```python
from build123d import *

# Parameters (mm, degrees)
SKETCH1_W                      = 15
SKETCH1_H                      = 5.8
CBORE_FOR_M3_SHCS1_D           = 3.2
CBORE_FOR_M3_SHCS1_CBORE_D     = 8
CBORE_FOR_M3_SHCS1_CBORE_DEPTH = 4.3
FILLET2_R                      = 4
FILLET3_R                      = 1


with BuildPart() as part:
    # Sketch1 → Revolve1 (revolve)
    with BuildSketch(Plane.XY, mode=Mode.PRIVATE) as revolve1_sk:
        with Locations((7.5, -2.9)):
            Rectangle(SKETCH1_W, SKETCH1_H)
    revolve(revolve1_sk.sketch.rotate(Axis((0, 0, 0), (0, -1, 0)), 180), axis=Axis((0, 0, 0), (0, -1, 0)))

    # CBORE for M3 SHCS1 (through all)
    with Locations(Plane(origin=(0, -5.8, 0), x_dir=(-1, 0, 0), z_dir=(0, -1, 0))):
        with Locations((0, 0)):
            CounterBoreHole(CBORE_FOR_M3_SHCS1_D / 2, CBORE_FOR_M3_SHCS1_CBORE_D / 2, CBORE_FOR_M3_SHCS1_CBORE_DEPTH)

    # Fillet2
    fillet2_edges = [part.edges().sort_by_distance(p)[0] for p in [
        (15, -5.8, 0),
    ]]
    fillet(fillet2_edges, radius=FILLET2_R)

    # Fillet3
    fillet3_edges = [part.edges().sort_by_distance(p)[0] for p in [
        (4, -5.8, 0),
    ]]
    fillet(fillet3_edges, radius=FILLET3_R)


solid = part.part
```
For this review, take the finished solid that the model builds, in its own axes (mm). A direction names the side the tool comes from. Coordinates: 2 decimals unless noted, no trailing zeros. Write each loop counter-clockwise with the first axis right and the second up, starting at its lowest first coordinate (ties: lowest second). Pieces come first, ordered by that corner, then holes. Notation, with made-up numbers: (19.25, 76.5) - (71.25, 76.5) arc R30 cw to (71.25, 103.5) - close; hole circle Ø4 at (89.25, -26). An arc over 180 degrees is marked (long way). Answer in a Markdown table with one row per item. Add a question column.
Q1. Tool access review of faces 1 (the flat face through (5, -5.8, 2)), 2 (the cylindrical face through (0.867, -3.173, 3.905)): name each direction out of +Z, -Z, +X, -X, +Y, -Y from which nothing blocks a thin tool from reaching the whole face with its end or side.
Q2. Draft analysis for pull direction Z (two halves, no side actions). For faces 3 (the flat face through (-2, -1.5, 0)), 4 (the cylindrical face through (-8.06, -0.89, -12.65)), 5 (the flat face through (3, 0, 0)), state which applies: +Z half, -Z half, draft (parallel to the pull), parting line (faces both ways), or undercut.
Q3. We need section D-D, the plane y = -2.3. State the section outline as (x, z) points, and give its area (3 significant figures).
Q4. We need section B-B, the plane z = 0. State the section outline as (x, y) points.
Q5. For P1, Ø1.5, axis at x = -11, y = -4.5, coming from the -Z side; P2, Ø2.5, axis at x = 0, z = 0, coming from the -Y side; P3, Ø2.5, axis at x = 2, z = -0.5, coming from the -Y side, all flat-tipped, find the tip position at first contact; note any pin that passes through.
Q6. We need section C-C, the plane y = -0.65. State the section outline as (x, z) points, and give its area (3 significant figures).
Q7. We need section A-A, the plane x = 0. State the section outline as (y, z) points.
Q8. For probe 1 along Z at (x, y) = (0, -0.25); probe 2 along Z at (x, y) = (0, -4.05); probe 3 along Z at (x, y) = (6.25, -3.3), list the stretches that pass through material, from the lowest coordinate up.
Answer list:
| question | item | result |
|---|---|---|
| 1 | face 1 | +Z, -Z, +X, -X, -Y |
| 1 | face 2 | -Y |
| 2 | face 3 | undercut |
| 2 | face 4 | parting line |
| 2 | face 5 | draft |
| 3 | outline | circle Ø29.94 at (0, 0); hole circle Ø8 at (0, 0) |
| 3 | area | 654 mm2 |
| 4 | outline | (-15, -1.8) arc R4 ccw to (-11, -5.8) - (-5, -5.8) arc R1 ccw to (-4, -4.8) - (-4, -1.5) - (-1.6, -1.5) - (-1.6, 0) - (-15, 0) - close; (1.6, -1.5) - (4, -1.5) - (4, -4.8) arc R1 ccw to (5, -5.8) - (11, -5.8) arc R4 ccw to (15, -1.8) - (15, 0) - (1.6, 0) - close |
| 5 | P1 | stops at z = -9.83 |
| 5 | P2 | passes through |
| 5 | P3 | stops at y = -1.5 |
| 6 | outline | circle Ø30 at (0, 0); hole circle Ø3.2 at (0, 0) |
| 6 | area | 699 mm2 |
| 7 | outline | (-5.8, -11) arc R4 ccw to (-1.8, -15) - (0, -15) - (0, -1.6) - (-1.5, -1.6) - (-1.5, -4) - (-4.8, -4) arc R1 ccw to (-5.8, -5) - close; (-5.8, 5) arc R1 ccw to (-4.8, 4) - (-1.5, 4) - (-1.5, 1.6) - (0, 1.6) - (0, 15) - (-1.8, 15) arc R4 ccw to (-5.8, 11) - close |
| 8 | probe 1 | z = -15 to -1.6, 1.6 to 15 |
| 8 | probe 2 | z = -14.31 to -4, 4 to 14.31 |
| 8 | probe 3 | z = -13.31 to 13.31 |
